Input: part model. Units: mm. Frame: model coordinates. A direction names the side the tool comes from. Give positions to 0.01 mm unless a question says otherwise; leave off trailing zeros. Order: outer loops, then holes, each group sorted by start corner. A loop starts at its lowest first (then second) coordinate and runs counter-clockwise, first axis right, second up. Notation, with made-up numbers: (13, 23) - (65, 23) arc R31 ccw to (65, 49) - close; hole circle Ø1 at (69, 57). An arc over 180 degrees is marked (long way). Answer in a Markdown table with one row per item. Add a question column.
1. Section query A-A on z = 3.75. Return loops of the section in (x, y).
2. Ray query, line 1 (X direction, y = 12, z = 1.75); line 2 (Y direction, x = 6.5, z = 3.25); line 3 (X direction, y = 6, z = 2). Return the intervals inside material, ascending. Write a range as [from, to].
3. Mould query, pull axis Y, two halves, no side actions, for faces 1 (the face through (18, 14, 1.6)), 2 (the face through (17, 16.21, 1.96)), 3 (the face through (21.952, 8.343, 4.058)), 4 (the face through (9.767, -8.579, 2.958)). Classes: released by +Y, released by -Y, zero draft, split by the parting line, or undercut.
4. Section query B-B on y = -14. Return loops of the section in (x, z).
5. Access query for faces 5 (the face through (21, 10, 4.4)), 6 (the face through (21.96, 8.33, 1.96)), 7 (the face through (16.78, 16.48, 3)), 8 (the face through (-3.81, 12.43, 2.96)), 9 (the face through (-1.5, -14.5, 3)). Directions: +Z, -Z, +X, -X, +Y, -Y. A direction counts if a zero-diameter tool reaches every point of the face in a straight line with its end or side. Return the directions, or none.
6. Contact query for flat-ended pins moving along their axis: pin 1 (1.5 mm diameter, centred on x = 17, y = -5.5, fed in from -Z); pin 2 (4 mm diameter, centred on x = 20, y = 10.5, fed in from -Z); pin 3 (3 mm diameter, centred on y = -1.5, z = 5.5, fed in from -X); pin 4 (1.2 mm diameter, centred on x = 17.5, y = 14.5, fed in from -Z). Output: stop coordinate, or through.
7. Section query C-C on x = -4. Return loops of the section in (y, z), and give its area (3 significant figures).
```python
from build123d import *

# Parameters (mm, degrees)
F1_DEPTH = 6
F2_R     = 1.8
F3_DEPTH = 2
F5_DEPTH = 3
F6_R     = 1.2
F8_DEPTH = 6.1
F9_R     = 1.3


# Not quite as in the source:
# - a feature names something its author has since deleted; it is built from what else it names


with BuildPart() as f1:
    # F0 (on Top) → F1 (new body)
    with BuildSketch(Plane.XY):
        with BuildLine():
            ThreePointArc((11, 6.9282032303), (11.3812706231, -6.2822511095), (0, -13))
            ThreePointArc((0, -13), (-1.5000000067, -14.4999999933), (-1.34e-08, -16))
            ThreePointArc((-1.34e-08, -16), (11.1120589721, -11.5118263277), (15.9900116293, -0.5652681616))
            Line((15.9900116293, -0.5652681616), (15.7964483902, -0.6871813851))
            Line((15.7964483902, -0.6871813851), (11, 6.9282032303))
        make_face()
        with BuildLine():
            ThreePointArc((-11.7246516205, 5.6153846154), (-0.7497687455, 12.9783607142), (11, 6.9282032303))
            Line((11, 6.9282032303), (6.2035516098, 14.5435878457))
            Line((6.2035516098, 14.5435878457), (6.3971148489, 14.6655010692))
            ThreePointArc((6.3971148489, 14.6655010692), (-5.582589802, 14.9944886909), (-14.4303404061, 6.9112427076))
            ThreePointArc((-14.4303404061, 6.9112427076), (-13.7254250594, 4.9104692687), (-11.7246516205, 5.6153846154))
        make_face()
        with BuildLine():
            Line((6.2035516098, 14.5435878457), (11, 6.9282032303))
            Line((11, 6.9282032303), (15.7964483902, -0.6871813851))
            Line((15.7964483902, -0.6871813851), (15.9900116293, -0.5652681616))
            ThreePointArc((15.9900116293, -0.5652681616), (13.5384615385, 8.5270193603), (6.3971148489, 14.6655010692))
            Line((6.3971148489, 14.6655010692), (6.2035516098, 14.5435878457))
        make_face()
        with BuildLine():
            ThreePointArc((6.3971148489, 14.6655010692), (13.5384615385, 8.5270193603), (15.9900116293, -0.5652681616))
            Line((15.9900116293, -0.5652681616), (21.2964483902, 2.77692023))
            Line((21.2964483902, 2.77692023), (11.7035516098, 18.0076894608))
            Line((11.7035516098, 18.0076894608), (6.3971148489, 14.6655010692))
        make_face()
    extrude(amount=F1_DEPTH)

    # F2 (on face) → F3 (join)
    with BuildSketch(Plane(origin=(16.5, 10.3923048454, 0), x_dir=(-0.53293871, 0.8461538462, 0), z_dir=(0.8461538462, 0.53293871, 0))):
        with Locations((0, 3)):
            Circle(F2_R)
    extrude(amount=F3_DEPTH)

    # F4 (on face) → F5 (join)
    with BuildSketch(Plane(origin=(18.1923076923, 11.4581822655, 0), x_dir=(-0.53293871, 0.8461538462, 0), z_dir=(0.8461538462, 0.53293871, 0))):
        with BuildLine():
            Line((-1.1313708499, 4.4), (1.1313708499, 4.4))
            ThreePointArc((1.1313708499, 4.4), (0, 4.8), (-1.1313708499, 4.4))
        make_face()
        with BuildLine():
            Line((-1.1313708499, 1.6), (1.1313708499, 1.6))
            ThreePointArc((1.1313708499, 1.6), (1.6242640687, 2.2242640687), (1.8, 3))
            ThreePointArc((1.8, 3), (1.6242640687, 3.7757359313), (1.1313708499, 4.4))
            Line((1.1313708499, 4.4), (-1.1313708499, 4.4))
            ThreePointArc((-1.1313708499, 4.4), (-1.8, 3), (-1.1313708499, 1.6))
        make_face()
        with BuildLine():
            Line((1.1313708499, 1.6), (5, 1.6))
            Line((5, 1.6), (5, 4.4))
            Line((5, 4.4), (1.1313708499, 4.4))
            ThreePointArc((1.1313708499, 4.4), (1.6242640687, 3.7757359313), (1.8, 3))
            ThreePointArc((1.8, 3), (1.6242640687, 2.2242640687), (1.1313708499, 1.6))
        make_face()
        with BuildLine():
            Line((-5, 1.6), (-1.1313708499, 1.6))
            ThreePointArc((-1.1313708499, 1.6), (-1.8, 3), (-1.1313708499, 4.4))
            Line((-1.1313708499, 4.4), (-5, 4.4))
            Line((-5, 4.4), (-5, 1.6))
        make_face()
        with BuildLine():
            ThreePointArc((-1.1313708499, 1.6), (0, 1.2), (1.1313708499, 1.6))
            Line((1.1313708499, 1.6), (-1.1313708499, 1.6))
        make_face()
    extrude(amount=F5_DEPTH)

    # F6
    f6_edges = [f1.edges().sort_by_distance(p)[0] for p in [
        (22.126232, 8.026821, 4.4),
        (22.126232, 8.026821, 1.6),
        (16.796845, 16.48836, 4.4),
        (16.796845, 16.48836, 1.6),
    ]]
    fillet(f6_edges, radius=F6_R)

    # F7 (on face) → F8 (cut)
    with BuildSketch(Plane.XY.offset(6)):
        with BuildLine():
            ThreePointArc((7.4891526037, 10.626033751), (9.4276549916, 8.9509396914), (11, 6.9282032303))
            Line((11, 6.9282032303), (12.6923076923, 7.9940806503))
            Line((12.6923076923, 7.9940806503), (10.0276141422, 12.2248498811))
            Line((10.0276141422, 12.2248498811), (7.4891526037, 10.626033751))
        make_face()
        with BuildLine():
            Line((12.6923076923, 7.9940806503), (11, 6.9282032303))
            ThreePointArc((11, 6.9282032303), (12.1451198736, 4.6363847183), (12.818539704, 2.1644952895))
            Line((12.818539704, 2.1644952895), (15.3570012424, 3.7633114195))
            Line((15.3570012424, 3.7633114195), (12.6923076923, 7.9940806503))
        make_face()
    extrude(amount=-F8_DEPTH, mode=Mode.SUBTRACT)

    # F9
    f9_edges = [f1.edges().sort_by_distance(p)[0] for p in [
        (7.489153, 10.626034, 3),
        (10.027614, 12.22485, 3),
        (12.81854, 2.164495, 3),
        (15.357001, 3.763311, 3),
    ]]
    fillet(f9_edges, radius=F9_R)


solid = f1.part
```
Answer:
| question | item | result |
|---|---|---|
| 1 | outline | (-14.43, 6.91) arc R1.5 ccw to (-11.72, 5.62) arc R13 cw to (6.82, 11.07) arc R1.3 ccw to (8.2, 11.07) - (8.93, 11.53) arc R1.3 cw to (10.72, 11.12) - (14.66, 4.86) arc R1.3 cw to (14.26, 3.07) - (13.53, 2.61) arc R1.3 ccw to (12.93, 1.37) arc R13 cw to (0, -13) arc R1.5 ccw to (0, -16) arc R16 ccw to (15.99, -0.57) - (21.3, 2.78) - (17.37, 9.01) - (19.06, 10.07) - (20.79, 7.34) - (23.32, 8.94) - (18.14, 17.17) - (15.6, 15.58) - (17.32, 12.84) - (15.63, 11.78) - (11.7, 18.01) - (6.4, 14.67) arc R16 ccw to start |
| 2 | line 1 | x = [-10.58, -5], [5, 15.49], [16.62, 21.4] |
| 2 | line 2 | y = [-14.62, -11.26], [11.26, 14.73] |
| 2 | line 3 | x = [-14.55, -11.53], [13.95, 19.27] |
| 3 | face 1 | zero draft |
| 3 | face 2 | released by +Y |
| 3 | face 3 | undercut |
| 3 | face 4 | undercut |
| 4 | outline | (-1.41, 0) - (7.75, 0) - (7.75, 6) - (-1.41, 6) - close |
| 5 | face 5 | +Z, +X |
| 5 | face 6 | -Z, +X |
| 5 | face 7 | +Z, -Z, +Y |
| 5 | face 8 | +Z, -Z |
| 5 | face 9 | +Z, -Z, -X |
| 6 | pin 1 | passes through |
| 6 | pin 2 | stops at z = 1.2 |
| 6 | pin 3 | stops at x = 12.65 |
| 6 | pin 4 | stops at z = 1.6 |
| 7 | outline | (12.37, 0) - (15.49, 0) - (15.49, 6) - (12.37, 6) - close |
| 7 | area | 18.7 mm² |
